Read the model definition and answer for the solid it produces. Units are mm, in the model's axes. A direction names the side the tool comes from. Give positions to 0.01 mm unless a question says otherwise; leave off trailing zeros. Order: outer loops, then holes, each group sorted by start corner. A loop starts at its lowest first (then second) coordinate and runs counter-clockwise, first axis right, second up. Notation, with made-up numbers: (-20.75, 6.5) - (-7.75, 6.5) arc R33 cw to (-7.75, 43.5) - close; hole circle Ø7 at (4, 26). An arc over 180 degrees is marked (long way). Write each question's results on one line, items separated by ' | '. Start each with the question number.
Q1. Flat-ended cylindrical pins translate along their axes: P1, Ø0.8, axis at x = 16, y = -8.5, coming from the +Z side; P2, Ø3, axis at x = 3, y = -13, coming from the +Z side. Find the tip coordinate at first contact, or state that the pin passes through.
Q2. Find section B-B on x = 3. Give the vertices of the cut face in (y, z).
Q3. A tool of negligible diameter and unlimited length cuts with its end or side. For faces 1 (the face through (0, -13, 6)), 2 (the face through (17.357, -13, 7)), from which of +Z, -Z, +X, -X, +Y, -Y can it reach the whole face along a straight path? Write none if from no direction.
Q4. Find the intervals of material crossed by line 1 along Z through (x, y) = (12.5, -13.25); line 2 along Z through (x, y) = (21.5, -13), in increasing order. Write a range as from..to.
Q5. For a pull along X with two mould halves and no side action, classify faces 3 (the face through (22.354, -13, 7)), 4 (the face through (15, -27.178, 2)), 5 (the face through (31.242, -13, 5)) as +X half, -X half, draft (parallel to the pull), parting line (faces both ways), or undercut.
Q6. Find section A-A on z = 8. Count the separate pieces of the cut face and the enclosed holes in it, and give its area (3 significant figures).
from build123d import *

# Parameters (mm, degrees)
F1_DEPTH = 27.178
F2_R     = 0.396875


with BuildPart() as f1:
    # F0 (on Front) → F1 (new body)
    with BuildSketch(Plane.XZ):
        Polygon((0, 0), (31.242, 0), (31.242, 11.1252), (30.0609, 11.1252), (30.0609, 2.2352), (26.588357, 2.2352), (26.588357, 11.1252), (25.826357, 11.1252), (25.826357, 2.2352), (22.353814, 2.2352), (22.353814, 11.1252), (21.591814, 11.1252), (21.591814, 2.2352), (18.119271, 2.2352), (18.119271, 11.1252), (17.357271, 11.1252), (17.357271, 2.2352), (13.884729, 2.2352), (13.884729, 11.1252), (13.122729, 11.1252), (13.122729, 2.2352), (9.650186, 2.2352), (9.650186, 11.1252), (8.888186, 11.1252), (8.888186, 2.2352), (5.415643, 2.2352), (5.415643, 11.1252), (4.653643, 11.1252), (4.653643, 2.2352), (1.1811, 2.2352), (1.1811, 11.1252), (0, 11.1252), align=None)
    extrude(amount=F1_DEPTH)

    # F2
    f2_edges = [f1.edges().sort_by_distance(p)[0] for p in [
        (1.1811, -13.589, 2.2352),
        (4.653643, -13.589, 2.2352),
        (5.415643, -13.589, 2.2352),
        (8.888186, -13.589, 2.2352),
        (9.650186, -13.589, 2.2352),
        (13.122729, -13.589, 2.2352),
        (13.884729, -13.589, 2.2352),
        (17.357271, -13.589, 2.2352),
        (18.119271, -13.589, 2.2352),
        (21.591814, -13.589, 2.2352),
        (22.353814, -13.589, 2.2352),
        (25.826357, -13.589, 2.2352),
        (26.588357, -13.589, 2.2352),
        (30.0609, -13.589, 2.2352),
    ]]
    fillet(f2_edges, radius=F2_R)


solid = f1.part
Working result:
1) P1: z = 2.24 | P2: z = 2.32
2) outline: (-27.18, 0) - (0, 0) - (0, 2.24) - (-27.18, 2.24) - close
3) face 1: +Z, -Z, -X, +Y, -Y | face 2: +Z, +Y, -Y
4) line 1: 0..2.24 | line 2: 0..2.38
5) face 3: undercut | face 4: draft | face 5: +X half
6) separate pieces: 8 | enclosed holes: 0 | area: 188 mm²
